Geometry check sheet. Reference: the model listing, model coordinates, mm. A direction names the side the tool comes from. Round coordinates to 2 decimals unless told otherwise and drop trailing zeros. Loops run counter-clockwise (first coordinate to the right, second up) from the corner with the lowest first, then second, coordinate; pieces in that order, holes last. Notation, with made-up numbers: (85, 2) - (93, 2) arc R18 ccw to (93, 9) - close; hole circle Ø6 at (81, 40.5). An arc over 180 degrees is marked (long way). Answer as CSV lines item,"result". Start each with the question number.
1) Access from +Z, -Z, +X, -X, +Y, -Y to the whole of each face (thin tool, end or side, straight path). Record for faces 4 (the cylindrical face through (-40, -16, -9)), 5 (the cylindrical face through (-124.88, 18.04, 5.5)), 6 (the flat face through (30, -16.13, -30)).
2) Draft check along Y on faces 1 (the cylindrical face through (14.278, 3.744, 22.395)), 2 (the cylindrical face through (32.79, 0.23, 25.14)), 3 (the flat face through (-27, -12.062, 1)). Enter one of: released by +Y, released by -Y, zero draft, split by the parting line, or undercut.
3) Cross-section at B-B on z = 0. Record the boundary of the cut face in (x, y), and give its area (3 significant figures).
4) Cross-section at A-A on x = 0. Record the boundary of the cut face in (y, z), and give its area (3 significant figures).
5) Cross-section at C-C on z = -32. Record the boundary of the cut face in (x, y).
6) Depth check by flat-ended pin: P1, Ø1, axis at x = 17, y = 4.5, coming from the -Z side; P2, Ø2, axis at x = -94.5, y = 15.5, coming from the +Z side; P3, Ø5, axis at x = 1.5, y = 5, coming from the +Z side. Enter the tip coordinate at first touch or a pass-through.
7) Cross-section at D-D on y = 1.5. Record the boundary of the cut face in (x, z).
8) Thickness scan on line 1 along Y through (x, z) = (43, 56.5); line 2 along Z through (x, y) = (0, -4); line 3 along X through (y, z) = (-14.5, 0). Record the ranges inside material, lowest first.
from build123d import *

# Parameters (mm, degrees)
F0_R     = 125
F1_DEPTH = 20
F2_R     = 26.56
F3_DEPTH = 20
F5_W     = 86.677861
F5_H     = 32.26
F7_W     = 7.9375
F7_H     = 41


with BuildPart() as f1:
    # F0 (on Front) → F1 (new body, symmetric)
    with BuildSketch(Plane.XZ):
        Circle(F0_R)
    extrude(amount=F1_DEPTH, both=True)

    # F2 (on Front) → F3 (cut, symmetric)
    with BuildSketch(Plane.XZ):
        Circle(F2_R)
    extrude(amount=F3_DEPTH, both=True, mode=Mode.SUBTRACT)

    # F5 (on Top) → F6 (revolve, cut)
    with BuildSketch(Plane.XY):
        with Locations((-84.65893, 0)):
            Rectangle(F5_W, F5_H)
    revolve(axis=Axis((0, 0, 0), (0, -1, 0)), mode=Mode.SUBTRACT)

    # F7 (on Right) → F8 (revolve, cut)
    with BuildSketch(Plane.YZ):
        with Locations((-16.03125, 20.5)):
            Rectangle(F7_W, F7_H)
    revolve(axis=Axis((0, -16.03125, 0), (0, 1, 0)), mode=Mode.SUBTRACT)


solid = f1.part
Answer block:
1,face 4,"-Y"
1,face 5,"+Y, -Y"
1,face 6,"none"
2,face 1,"zero draft"
2,face 2,"undercut"
2,face 3,"released by -Y"
3,outline,"(-125, -20) - (-41, -20) - (-41, -12.06) - (-26.56, -12.06) - (-26.56, 20) - (-125, 20) - (-125, 16.13) - (-41.32, 16.13) - (-41.32, -16.13) - (-125, -16.13) - close; (26.56, -12.06) - (41, -12.06) - (41, -20) - (125, -20) - (125, -16.13) - (41.32, -16.13) - (41.32, 16.13) - (125, 16.13) - (125, 20) - (26.56, 20) - close"
3,area,"2,250 mm^2"
4,outline,"(-20, -125) - (-16.13, -125) - (-16.13, -41.32) - (16.13, -41.32) - (16.13, -125) - (20, -125) - (20, -26.56) - (-12.06, -26.56) - (-12.06, -41) - (-20, -41) - close; (-20, 41) - (-12.06, 41) - (-12.06, 26.56) - (20, 26.56) - (20, 125) - (16.13, 125) - (16.13, 41.32) - (-16.13, 41.32) - (-16.13, 125) - (-20, 125) - close"
4,area,"2,250 mm^2"
5,outline,"(-120.83, -20) - (-25.63, -20) - (-25.63, -12.06) - (25.63, -12.06) - (25.63, -20) - (120.83, -20) - (120.83, -16.13) - (26.14, -16.13) - (26.14, 16.13) - (120.83, 16.13) - (120.83, 20) - (-120.83, 20) - (-120.83, 16.13) - (-26.14, 16.13) - (-26.14, -16.13) - (-120.83, -16.13) - close"
6,P1,"stops at z = -37.88"
6,P2,"stops at z = 82.71"
6,P3,"stops at z = 41.32"
7,outline,"circle Ø82.64 at (0, 0); hole circle Ø53.12 at (0, 0)"
8,line 1,"y = -20 to -16.13, 16.13 to 20"
8,line 2,"z = -41.32 to -26.56, 26.56 to 41.32"
8,line 3,"x = -41.32 to -41, 41 to 41.32"
